Design review of the part built by this model. Coordinates are the model's own, in mm. A direction names the side the tool comes from. Coordinates: 2 decimals unless noted, no trailing zeros. Loops run counter-clockwise (first coordinate to the right, second up) from the corner with the lowest first, then second, coordinate; pieces in that order, holes last. Notation, with made-up numbers: (85.5, -15) - (124.5, -15) arc R27 ccw to (124.5, 6) - close; hole circle Ø5 at (32.5, 82.25). An arc over 180 degrees is marked (long way). Return JSON: item names as keys, results as strings. Group by question number.
from build123d import *

# Parameters (mm, degrees)
F0_W        = 555
F0_H        = 305
F1_DEPTH    = 50
F2_W        = 595
F2_H        = 345
F2_W_2      = 555
F2_H_2      = 305
F3_DEPTH    = 1.5
F4_T        = 1.5
F4_T3_DEPTH = 308
F4_T5_DEPTH = 558


# Not quite as in the source:
# - a shell that OpenCascade refuses in one call is made with other operations: the cavity is built on its own and cut out


with BuildPart() as f1:
    # F0 (on Top) → F1 (new body)
    with BuildSketch(Plane.XY):
        Rectangle(F0_W, F0_H)
    extrude(amount=-F1_DEPTH)

    # F2 (on face) → F3 (join)
    with BuildSketch(Plane.XY):
        Rectangle(F2_W, F2_H)
        Rectangle(F2_W_2, F2_H_2, mode=Mode.SUBTRACT)
        Rectangle(F2_W_2, F2_H_2)
    extrude(amount=F3_DEPTH)

    # F4: shell of thickness 1.5, made by hand


with BuildPart() as f4_core1:
    # F4_t2: copy of F1
    add(f1.part)

    # the walls: a layer under each face that stays
    f4_faces = [f4_core1.faces().sort_by_distance(p)[0] for p in [
        (-297.5, 0, 0.75),
        (0, 172.5, 0.75),
        (0, -172.5, 0.75),
        (-277.6666666667, -161, 0),
        (297.5, 0, 0.75),
        (-277.5, 0, -25),
        (0, -152.5, -25),
        (277.5, 0, -25),
        (0, 152.5, -25),
        (0, 0, -50),
    ]]
    thicken(f4_faces, amount=-F4_T, mode=Mode.SUBTRACT)

    # F4_s4 → F4_t3 (cut)
    with BuildSketch(Plane.XZ.offset(-154)):
        Polygon((-277.515, -0.015), (-277.5, 1.5), (-276, 1.5), (-276, 0), align=None)
        Polygon((277.515, -0.015), (277.5, 1.5), (276, 1.5), (276, 0), align=None)
    extrude(amount=F4_T3_DEPTH, mode=Mode.SUBTRACT)

    # F4_s6 → F4_t5 (cut)
    with BuildSketch(Plane.YZ.offset(-279)):
        Polygon((-152.515, -0.015), (-152.5, 1.5), (-151, 1.5), (-151, 0), align=None)
        Polygon((152.515, -0.015), (152.5, 1.5), (151, 1.5), (151, 0), align=None)
    extrude(amount=F4_T5_DEPTH, mode=Mode.SUBTRACT)


with BuildPart() as f1_1:
    add(f1.part)

    # what is left inside the walls is the cavity
    f4_cavity = [f4_core1.part.solids().sort_by_distance(p)[0] for p in [
        (0, -50.333333, -48.485),
    ]]
    add(f4_cavity, mode=Mode.SUBTRACT)


solid = f1_1.part
Item 1: Add section A-A (z = -34). State the section outline as (x, y) points, then the cut area to 3 significant figures.
Item 2: For faces 4 (the face through (277.5, -2, -25)), 5 (the face through (-4, -151, -23)), 6 (the face through (-4, -152.5, -25)), 7 (the face through (-23, -153, 1.5)), 8 (the face through (-4, 2, -50)), list the 3-axis set-ups (+Z, -Z, +X, -X, +Y, -Y) from which the entire face can be reached by the end or side of a thin tool; tool diameter is ignored.
Item 3: For P1, Ø12, axis at y = -1, z = -19.5, coming from the +X side; P2, Ø5, axis at x = 0, z = -24.5, coming from the -Y side; P3, Ø4, axis at x = 24.5, y = -26.5, coming from the +Z side, all flat-tipped, find the tip position at first contact; note any pin that passes through.
Item 4: Add section C-C (y = 15). State the section outline as (x, z) points.
Item 5: Draft analysis for pull direction X (two halves, no side actions). For faces 1 (the face through (-277.5, -2, -25)), 2 (the face through (276, 2, -23)), 3 (the face through (-4, 152.5, -25)), state which applies: pulls with the +X half, pulls with the -X half, needs draft (parallel to the pull), parting line crosses it, or undercut.
Item 6: Add section B-B (x = 132). State the section outline as (y, z) points.
Item 7: To check wall thickness, follow line 1 (X direction, y = 10, z = -6.5); line 2 (Y direction, x = -22, z = -18); line 3 (Z direction, x = 140.5, y = 153.5). State the ranges of each line that lie inside material, in increasing order. Write a range as from..to.
Answers below:
{
 "1": {"outline": "(-277.5, -152.5) - (277.5, -152.5) - (277.5, 152.5) - (-277.5, 152.5) - close; hole (-276, -151) - (276, -151) - (276, 151) - (-276, 151) - close", "area": "2,570 mm^2"},
 "2": {"face 4": "-Z, +X, +Y, -Y", "face 5": "+Z", "face 6": "-Z, +X, -X, -Y", "face 7": "+Z, +X, -X, +Y, -Y", "face 8": "-Z, +X, -X, +Y, -Y"},
 "3": {"P1": "stops at x = 277.5", "P2": "stops at y = -152.5", "P3": "stops at z = -48.5"},
 "4": {"outline": "(-297.5, 0) - (-277.5, 0) - (-277.5, -50) - (277.5, -50) - (277.5, 0) - (297.5, 0) - (297.5, 1.5) - (276, 1.5) - (276, -48.5) - (-276, -48.5) - (-276, 1.5) - (-297.5, 1.5) - close"},
 "5": {"face 1": "pulls with the -X half", "face 2": "undercut", "face 3": "needs draft"},
 "6": {"outline": "(-172.5, 0) - (-152.5, 0) - (-152.5, -50) - (152.5, -50) - (152.5, 0) - (172.5, 0) - (172.5, 1.5) - (151, 1.5) - (151, -48.5) - (-151, -48.5) - (-151, 1.5) - (-172.5, 1.5) - close"},
 "7": {"line 1": "x = -277.5..-276, 276..277.5", "line 2": "y = -152.5..-151, 151..152.5", "line 3": "z = 0..1.5"}
}
